```python
from build123d import *

# Parameters (mm, degrees)
BOSS_EXTRUDE1_DEPTH = 203.2
FILLET1_R           = 7.62
SKETCH2_R           = 61.722
BOSS_EXTRUDE2_DEPTH = 147.1422
FILLET2_R           = 7.62
SKETCH4_R           = 61.722
CUT_EXTRUDE2_DEPTH  = 121.7422
SKETCH6_R           = 50.8
CUT_EXTRUDE3_DEPTH  = 101.6
SKETCH5_R           = 50.8
CUT_EXTRUDE4_DEPTH  = 101.6
BOSS_EXTRUDE3_START = 25.4
SKETCH7_W           = 401.32
SKETCH7_H           = 203.2
SKETCH7_R           = 61.722
BOSS_EXTRUDE3_DEPTH = 25.4
FILLET3_R           = 7.62


with BuildPart() as part:
    # Sketch1 → Boss-Extrude1 (new body)
    with BuildSketch(Plane.XY):
        Polygon((129.54, 113.962405063), (-129.54, 113.962405063), (-200.66, -267.037594937), (200.66, -267.037594937), align=None)
    extrude(amount=BOSS_EXTRUDE1_DEPTH)

    # Fillet1
    fillet1_edges = [part.edges().sort_by_distance(p)[0] for p in [
        (-165.1, -76.537594937, 203.2),
        (165.1, -76.537594937, 203.2),
        (-165.1, -76.537594937, 0),
        (0, 113.962405063, 0),
        (165.1, -76.537594937, 0),
        (0, 113.962405063, 203.2),
        (-129.54, 113.962405063, 101.6),
        (129.54, 113.962405063, 101.6),
    ]]
    fillet(fillet1_edges, radius=FILLET1_R)

    # Sketch2 → Boss-Extrude2 (add)
    with BuildSketch(Plane(origin=(0, 113.962405063, 0), x_dir=(1, 0, 0), z_dir=(0, 1, 0))):
        with Locations((1.290779411, -101.591800302)):
            Circle(SKETCH2_R)
    extrude(amount=BOSS_EXTRUDE2_DEPTH)

    # Fillet2
    fillet2_edges = [part.edges().sort_by_distance(p)[0] for p in [
        (-60.431220589, 261.104605063, 101.591800302),
    ]]
    fillet(fillet2_edges, radius=FILLET2_R)

    # Sketch4 → Cut-Extrude2 (cut)
    with BuildSketch(Plane(origin=(0, -267.037594937, 0), x_dir=(-1, 0, 0), z_dir=(0, -1, 0))):
        with Locations(Location((100.33, -101.6, 0), (0, 0, 90))):
            Circle(SKETCH4_R)
        with Locations(Location((-100.33, -101.6, 0), (0, 0, 90))):
            Circle(SKETCH4_R)
    extrude(amount=-CUT_EXTRUDE2_DEPTH, mode=Mode.SUBTRACT)

    # Sketch6 → Cut-Extrude3 (cut)
    with BuildSketch(Plane(origin=(145.73492962, 27.203853529, 0), x_dir=(0, 0, -1), z_dir=(0.9830202487654599, 0.18349711310288594, 0))):
        with Locations(Location((-101.6, -12.052084845, 0), (0, 0, 90))):
            Circle(SKETCH6_R)
    extrude(amount=-CUT_EXTRUDE3_DEPTH, mode=Mode.SUBTRACT)

    # Sketch5 → Cut-Extrude4 (cut)
    with BuildSketch(Plane(origin=(-145.73492962, 27.203853529, 0), x_dir=(0, 0, 1), z_dir=(-0.98302024876546, 0.18349711310288583, 0))):
        with Locations(Location((101.6, -12.052084845, 0), (0, 0, 270))):
            Circle(SKETCH5_R)
    extrude(amount=-CUT_EXTRUDE4_DEPTH, mode=Mode.SUBTRACT)

    # Sketch7 → Boss-Extrude3 (add)
    with BuildSketch(Plane.XZ.offset(267.037594937).offset(BOSS_EXTRUDE3_START)):
        with Locations((0, 101.6)):
            Rectangle(SKETCH7_W, SKETCH7_H)
        with Locations(Location((-100.33, 101.6, 0), (0, 0, 270))):
            Circle(SKETCH7_R, mode=Mode.SUBTRACT)
        with Locations(Location((100.33, 101.6, 0), (0, 0, 270))):
            Circle(SKETCH7_R, mode=Mode.SUBTRACT)
    extrude(amount=-BOSS_EXTRUDE3_DEPTH)

    # Fillet3
    fillet3_edges = [part.edges().sort_by_distance(p)[0] for p in [
        (-200.66, -279.737594937, 0),
        (200.66, -279.737594937, 203.2),
        (200.66, -279.737594937, 0),
        (-200.66, -279.737594937, 203.2),
    ]]
    fillet(fillet3_edges, radius=FILLET3_R)


solid = part.part
```
Read the model definition and answer for the solid it produces. Units are mm, in the model's axes. A direction names the side the tool comes from. Coordinates: 2 decimals unless noted, no trailing zeros. Loops run counter-clockwise (first coordinate to the right, second up) from the corner with the lowest first, then second, coordinate; pieces in that order, holes last. Notation, with made-up numbers: (76.25, -21) - (115.25, -21) arc R28 ccw to (115.25, 13) - close; hole circle Ø3 at (38.5, 78.5). An arc over 180 degrees is marked (long way). Answer in a Markdown table with one row per item.
1. Find section B-B, the plane y = -254. Count the separate pieces of the cut face and the enclosed holes in it, then the cut area to 3 significant figures.
Conclusion:
| item | result |
|---|---|
| separate pieces | 1 |
| enclosed holes | 2 |
| area | 56,600 mm² |
2. Given pin 1 (1.5 mm diameter, centred on x = 134, z = 99.5, fed in from -Y); pin 2 (5 mm diameter, centred on y = 33, z = 155.5, fed in from +X); pin 3 (12 mm diameter, centred on y = -187, z = 100, fed in from +X), each flat-ended and moving along its own axis, determine where each tip first touches the part or whether it passes through.
Conclusion:
| item | result |
|---|---|
| pin 1 | stops at y = -145.3 |
| pin 2 | stops at x = 145.12 |
| pin 3 | stops at x = 186.84 |
3. Determine the mould class of faces 1 (the face through (29.77, 182.75, 156.35)), 2 (the face through (-97.495, 12.666, 151.968)), 3 (the face through (99.922, -0.336, 151.968)), 4 (the face through (2, 113.962, 38)) for opening direction Z: +Z half, -Z half, draft (parallel to the pull), parting line (faces both ways), or undercut.
Conclusion:
| item | result |
|---|---|
| face 1 | parting line |
| face 2 | undercut |
| face 3 | undercut |
| face 4 | draft |
4. Find section A-A, the plane z = 31. Write down the section's boundary in (x, y).
Conclusion:
| item | result |
|---|---|
| outline | (-200.66, -292.44) - (200.66, -292.44) - (200.66, -267.04) - (130.7, 107.74) arc R7.62 ccw to (123.21, 113.96) - (-123.21, 113.96) arc R7.62 ccw to (-130.7, 107.74) - (-200.66, -267.04) - close |
5. Which of the six approach directions +Z, -Z, +X, -X, +Y, -Y give full straight-line access (tool end or side, diameter ignored) to faces 5 (the face through (48.202, -3.986, 102.311)), 6 (the face through (62.8, -219.9, 150.6)), 7 (the face through (-164.03, -82.67, 2.29))?
Conclusion:
| item | result |
|---|---|
| face 5 | none |
| face 6 | -Y |
| face 7 | -Z, -X, +Y |
6. Straight lines are drawn through the part: line 1 (X direction, y = -182, z = 101.6); line 2 (X direction, y = -215.5, z = 101.6); line 3 (Y direction, x = 64, z = 41.5). For each, find the intervals that lie inside material, in ascending order.
Conclusion:
| item | result |
|---|---|
| line 1 | x = -184.79 to -162.05, -38.61 to 38.61, 162.05 to 184.79 |
| line 2 | x = -191.04 to -162.05, -38.61 to 38.61, 162.05 to 191.04 |
| line 3 | y = -292.44 to 113.96 |
